Geometry check sheet. Reference: drawing and pictorial views, mm from the part's lowest x, y, z. Round coordinates to 2 decimals unless told otherwise and drop trailing zeros. Order: outer loops, then holes, each group sorted by start corner. A loop starts at its lowest first (then second) coordinate and runs counter-clockwise, first axis right, second up.
Q1. Scan lines: probe 1 along Z at (x, y) = (14, 2.4); probe 2 along Z at (x, y) = (15.5, 3.95); probe 3 along X at (y, z) = (2.8, 6). Record each from-to range of solid material in increasing order.
Q2. Cross-section at C-C on y = 2.35. Record the cut outline in (x, z), then the cut area to 3 significant figures.
Q3. Cross-section at A-A on z = 43. Record the cut outline in (x, y), then the cut area to 3 significant figures.
Q4. Mould release check, pull along X, two halves, no side actions. Record for the marked faces 1, 2 and 3: +X half, -X half, draft (parallel to the pull), parting line (faces both ways), or undercut.
Q5. Cross-section at B-B on x = 14.25. Record the cut outline in (y, z).
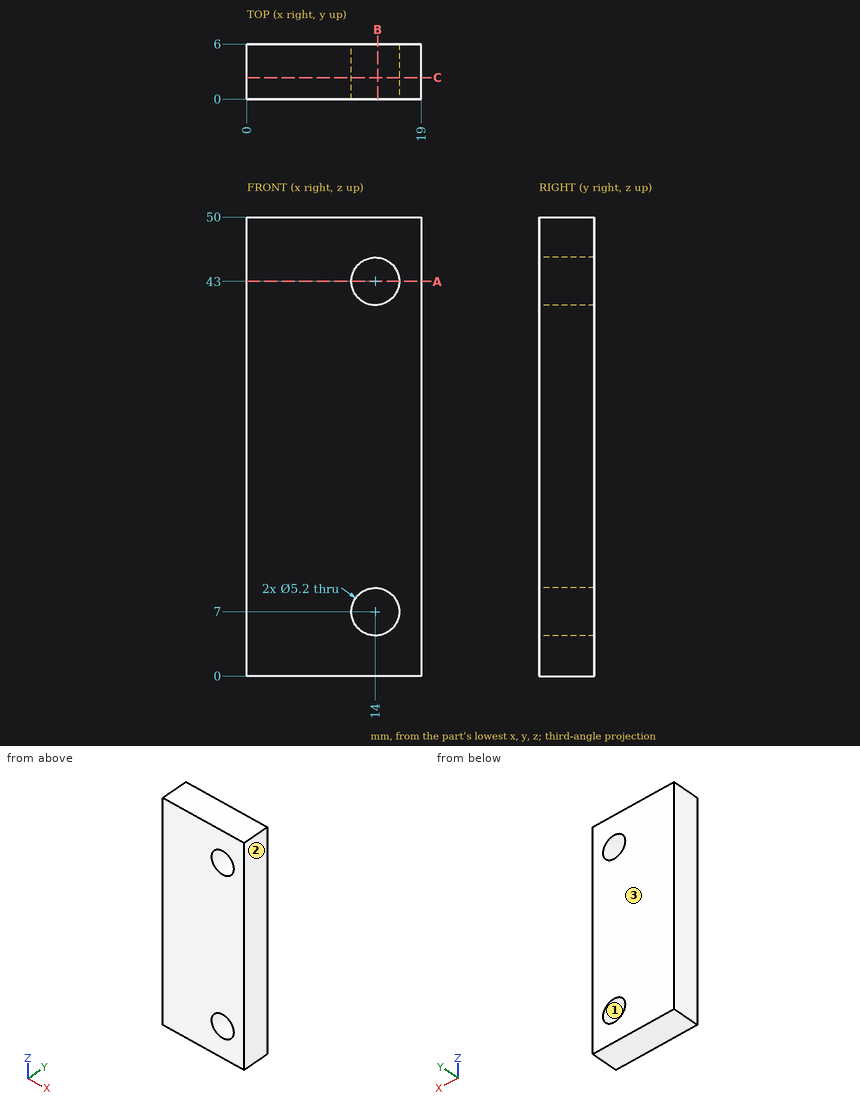
Results found:
1. probe 1: z = 0 to 4.4, 9.6 to 40.4, 45.6 to 50
1. probe 2: z = 0 to 4.88, 9.12 to 40.88, 45.12 to 50
1. probe 3: x = 0 to 11.6, 16.4 to 19
2. outline: (0, 0) - (19, 0) - (19, 50) - (0, 50) - close; hole circle Ø5.2 at (14, 7); hole circle Ø5.2 at (14, 43)
2. area: 908 mm2
3. outline: (0, 0) - (11.4, 0) - (11.4, 6) - (0, 6) - close; (16.6, 0) - (19, 0) - (19, 6) - (16.6, 6) - close
3. area: 82.8 mm2
4. face 1: undercut
4. face 2: +X half
4. face 3: draft
5. outline: (0, 0) - (6, 0) - (6, 4.41) - (0, 4.41) - close; (0, 9.59) - (6, 9.59) - (6, 40.41) - (0, 40.41) - close; (0, 45.59) - (6, 45.59) - (6, 50) - (0, 50) - close
